```python
from build123d import *

# Parameters (mm, degrees)
ESQUISSE1_W             = 52.2
ESQUISSE1_H             = 80
BOSS_EXTRU_2_DEPTH      = 22
ESQUISSE3_W             = 48.72
ESQUISSE3_H             = 72.8776
ENL_V_MAT_EXTRU_1_DEPTH = 5
CONG_1_R                = 10
BOSS_EXTRU_4_DEPTH      = 5
ESQUISSE2_R             = 16
ENL_V_MAT_EXTRU_3_DEPTH = 93.647092521
ENL_V_MAT_EXTRU_5_DEPTH = 2
ESQUISSE8_W             = 10.19
ESQUISSE8_H             = 3.5612
ENL_V_MAT_EXTRU_6_DEPTH = 4
CONG_3_R                = 2
ESQUISSE9_W             = 10.1
ESQUISSE9_H             = 80
BOSS_EXTRU_5_DEPTH      = 2.5
CONG_4_R                = 5


with BuildPart() as part:
    # Esquisse1 → Boss.-Extru.2 (new body)
    with BuildSketch(Plane.XY):
        with Locations((-15.124795362, -42.006460905)):
            Rectangle(ESQUISSE1_W, ESQUISSE1_H)
    extrude(amount=BOSS_EXTRU_2_DEPTH)

    # Esquisse3 → Enlèv. mat.-Extru.1 (cut)
    with BuildSketch(Plane.XY.offset(22)):
        with Locations((-15.124795362, -42.006460905)):
            Rectangle(ESQUISSE3_W, ESQUISSE3_H)
    extrude(amount=-ENL_V_MAT_EXTRU_1_DEPTH, mode=Mode.SUBTRACT)

    # Congé1
    cong_1_edges = [part.edges().sort_by_distance(p)[0] for p in [
        (-39.484795362, -78.445260905, 19.5),
        (-39.484795362, -5.567660905, 19.5),
        (9.235204638, -5.567660905, 19.5),
        (9.235204638, -78.445260905, 19.5),
    ]]
    fillet(cong_1_edges, radius=CONG_1_R)

    # Esquisse5 → Boss.-Extru.4 (add)
    with BuildSketch(Plane.XY.offset(17)):
        with BuildLine():
            Line((-35.624795362, -68.445260905), (-35.624795362, -76.006460905))
            Line((-35.624795362, -76.006460905), (-29.484795362, -76.006460905))
            Line((-29.484795362, -76.006460905), (-29.484795362, -78.445260905))
            ThreePointArc((-29.484795362, -78.445260905), (-36.555863174, -75.516328717), (-39.484795362, -68.445260905))
            Line((-39.484795362, -68.445260905), (-39.484795362, -15.567660905))
            ThreePointArc((-39.484795362, -15.567660905), (-36.555863174, -8.496593093), (-29.484795362, -5.567660905))
            Line((-29.484795362, -5.567660905), (-0.764795362, -5.567660905))
            ThreePointArc((-0.764795362, -5.567660905), (6.30627245, -8.496593093), (9.235204638, -15.567660905))
            Line((9.235204638, -15.567660905), (9.235204638, -68.445260905))
            ThreePointArc((9.235204638, -68.445260905), (6.30627245, -75.516328717), (-0.764795362, -78.445260905))
            Line((-0.764795362, -78.445260905), (-0.764795362, -76.006460905))
            Line((-0.764795362, -76.006460905), (5.375204638, -76.006460905))
            Line((5.375204638, -76.006460905), (5.375204638, -68.445260905))
            Line((5.375204638, -68.445260905), (5.375204638, -15.567660905))
            Line((5.375204638, -15.567660905), (5.375204638, -8.006460905))
            Line((5.375204638, -8.006460905), (-35.624795362, -8.006460905))
            Line((-35.624795362, -8.006460905), (-35.624795362, -15.567660905))
            Line((-35.624795362, -15.567660905), (-35.624795362, -68.445260905))
        make_face()
    extrude(amount=BOSS_EXTRU_4_DEPTH)

    # Esquisse2 → Enlèv. mat.-Extru.3 (cut, through all)
    with BuildSketch(Plane.XZ.offset(82.006460905)):
        with Locations((-15.124795362, 0)):
            Circle(ESQUISSE2_R)
    extrude(amount=-ENL_V_MAT_EXTRU_3_DEPTH, mode=Mode.SUBTRACT)

    # Esquisse7 → Enlèv. mat.-Extru.5 (cut)
    with BuildSketch(Plane.XY.offset(17)):
        Polygon((-35.624795362, -8.006460905), (5.375204638, -8.006460905), (5.375204638, -76.006460905), (-0.764795362, -76.006460905), (-0.764795362, -78.445260905), (-29.484795362, -78.445260905), (-29.484795362, -76.006460905), (-35.624795362, -76.006460905), align=None)
    extrude(amount=-ENL_V_MAT_EXTRU_5_DEPTH, mode=Mode.SUBTRACT)

    # Esquisse8 → Enlèv. mat.-Extru.6 (cut)
    with BuildSketch(Plane.XY.offset(22)):
        with Locations((-15.124795362, -80.225860905)):
            Rectangle(ESQUISSE8_W, ESQUISSE8_H)
    extrude(amount=-ENL_V_MAT_EXTRU_6_DEPTH, mode=Mode.SUBTRACT)

    # Congé3
    cong_3_edges = [part.edges().sort_by_distance(p)[0] for p in [
        (-20.219795362, -80.225860905, 18),
        (-10.029795362, -80.225860905, 18),
    ]]
    fillet(cong_3_edges, radius=CONG_3_R)

    # Esquisse9 → Boss.-Extru.5 (add)
    with BuildSketch(Plane(origin=(0, 0, 0), x_dir=(-1, 0, 0), z_dir=(0, 0, -1))):
        with Locations((36.174795362, -42.006460905)):
            Rectangle(ESQUISSE9_W, ESQUISSE9_H)
        with Locations((-5.925204638, -42.006460905)):
            Rectangle(ESQUISSE9_W, ESQUISSE9_H)
    extrude(amount=BOSS_EXTRU_5_DEPTH)

    # Congé4
    cong_4_edges = [part.edges().sort_by_distance(p)[0] for p in [
        (-41.224795362, -2.006460905, 9.75),
        (10.975204638, -2.006460905, 9.75),
        (10.975204638, -82.006460905, 9.75),
        (-41.224795362, -82.006460905, 9.75),
    ]]
    fillet(cong_4_edges, radius=CONG_4_R)


solid = part.part
```
Input: part model. Units: mm. Frame: model coordinates. A direction names the side the tool comes from. Give positions to 0.01 mm unless a question says otherwise; leave off trailing zeros. Write each loop counter-clockwise with the first axis right and the second up, starting at its lowest first coordinate (ties: lowest second). Pieces come first, ordered by that corner, then holes. Notation, with made-up numbers: (42.25, 29.5) - (49.25, 29.5) arc R18 cw to (49.25, 34.5) - close; hole circle Ø2 at (81.25, -1.75). An arc over 180 degrees is marked (long way). Write item = value, one per line. Start each with the question number.
1) Cut plane D-D (z = 9.5). Return loops of the section in (x, y).
2) Draft query along X for faces 1 (the face through (9.55, -3.51, 9.58)), 2 (the face through (-15, -80, 18)), 3 (the face through (-10.1, -82.006, 15.4)), 4 (the face through (-15, -8.006, 18)). Return one class per face: pulls with the +X half, pulls with the -X half, needs draft (parallel to the pull), parting line crosses it, or undercut.
3) Pin query (flat end, axial travel): pin 1 (2 mm diameter, centred on x = -3.5, y = -64.5, fed in from -Z); pin 2 (4 mm diameter, centred on x = -14.5, y = -80.5, fed in from +Z); pin 3 (10 mm diameter, centred on x = -7, y = -11, fed in from -Z); pin 4 (10 mm diameter, centred on x = -23.5, z = 5.5, fed in from +Y). Return the tip coordinate at first contact, or that it passes through.
4) Reachability of faces 5 (the face through (-10.6, -80.2, 18.6)), 6 (the face through (0.875, -43, -1)), 7 (the face through (9.55, -80.5, 9.92)), 8 (the face through (-35.625, -42, 18)) from +Z, -Z, +X, -X, +Y, -Y: full face, straight path, thin tool, end or side. Return the list, or none.
5) Cut plane C-C (x = -2). Return loops of the section in (y, z), and give its area (3 significant figures).
6) Material intervals for L1, parallel to Y at x = -8, z = 18.75; L2, parallel to Y at x = 0, z = 15.5; L3, parallel to X at y = -28, z = 16.25, sorted ascending. Write a range as [from, to].
7) Cut plane A-A (y = -44). Return loops of the section in (x, z), and give its area (3 significant figures).
8) Cut plane B-B (z = 5.5). Return loops of the section in (x, y), and give its area (3 significant figures).
Answers follow:
q1.outline = (-41.22, -77.01) arc R5 ccw to (-36.22, -82.01) - (-28, -82.01) - (-28, -2.01) - (-36.22, -2.01) arc R5 ccw to (-41.22, -7.01) - close; (-2.25, -82.01) - (5.98, -82.01) arc R5 ccw to (10.98, -77.01) - (10.98, -7.01) arc R5 ccw to (5.98, -2.01) - (-2.25, -2.01) - close
q2.face_1 = pulls with the +X half
q2.face_2 = undercut
q2.face_3 = needs draft
q2.face_4 = undercut
q3.pin_1 = 9.83
q3.pin_2 = 18
q3.pin_3 = 9.15
q3.pin_4 = through
q4.face_5 = +Z, -Y
q4.face_6 = -Z, +Y, -Y
q4.face_7 = +Z, -Z, +X, -Y
q4.face_8 = +Z
q5.outline = (-82.01, 9.15) - (-2.01, 9.15) - (-2.01, 22) - (-8.01, 22) - (-8.01, 15) - (-78.45, 15) - (-78.45, 22) - (-82.01, 22) - close
q5.area = 535 mm^2
q6.L1 = [-82.01, -78.45], [-8.01, -2.01]
q6.L2 = [-82.01, -76.01], [-8.01, -2.01]
q6.L3 = [-41.22, -35.62], [5.38, 10.98]
q7.outline = (-41.22, -2.5) - (-31.12, -2.5) - (-31.12, 0) arc R16 cw to (-20.69, 15) - (-35.62, 15) - (-35.62, 22) - (-41.22, 22) - close; (-9.56, 15) arc R16 cw to (0.88, 0) - (0.88, -2.5) - (10.98, -2.5) - (10.98, 22) - (5.38, 22) - (5.38, 15) - close
q7.area = 517 mm^2
q8.outline = (-41.22, -77.01) arc R5 ccw to (-36.22, -82.01) - (-30.15, -82.01) - (-30.15, -2.01) - (-36.22, -2.01) arc R5 ccw to (-41.22, -7.01) - close; (-0.1, -82.01) - (5.98, -82.01) arc R5 ccw to (10.98, -77.01) - (10.98, -7.01) arc R5 ccw to (5.98, -2.01) - (-0.1, -2.01) - close
q8.area = 1,750 mm^2
